from build123d import *

# Parameters (mm, degrees)
F1_DEPTH = 30
F2_T     = -5


with BuildPart() as f1:
    # F0 (on Top) → F1 (new body)
    with BuildSketch(Plane.XY):
        Polygon((0, 50), (-50, 0), (0, 0), align=None)
    extrude(amount=F1_DEPTH)

    # F2
    f2_openings = [f1.faces().sort_by_distance(p)[0] for p in [
        (-16.666667, 16.666667, 30),
    ]]
    offset(amount=F2_T, openings=f2_openings)


solid = f1.part
Verification items for the finished model (mm, model axes). A direction names the side the tool comes from. Coordinates: 2 decimals unless noted, no trailing zeros. Order: outer loops, then holes, each group sorted by start corner. A loop starts at its lowest first (then second) coordinate and runs counter-clockwise, first axis right, second up. Notation, with made-up numbers: (32.25, 29.25) -> (36.25, 29.25) arc R20 ccw to (36.25, 59.25) -> close; hole circle Ø3 at (33, 49). An arc over 180 degrees is marked (long way). Use CSV: the item, a comma, the result in double quotes. Start each with the question number.
Q1. Draft check along X on faces 1 (the flat face through (-14, 14, 5)), 2 (the flat face through (-23, 21, 30)), 3 (the flat face through (-25, 25, 15)). Enter one of: +X half, -X half, draft (parallel to the pull), parting line (faces both ways), or undercut.
Q2. Section check B-B, the plane x = -35.5. Record the cut outline in (y, z).
Q3. Section check A-A, the plane z = 28. Record the cut outline in (x, y), and give its area (3 significant figures).
Q4. Depth check by flat-ended pin: P1, Ø12.5, axis at y = 17, z = 19.5, coming from the -X side; P2, Ø7.5, axis at x = -14, z = 22.5, coming from the +Y side; P3, Ø2, axis at x = -28.5, z = 26.5, coming from the +Y side. Enter the tip coordinate at first touch or a pass-through.
Q5. Tool access check on faces 4 (the flat face through (-25, 0, 15)), 5 (the flat face through (-5, 21, 17)). Record the directions out of +Z, -Z, +X, -X, +Y, -Y that give a thin tool (end or side, any length) a straight path to the whole face; none if there is none.
Q6. Section check D-D, the plane z = 4.25. Record the cut outline in (x, y), and give its area (3 significant figures).
Q7. Section check C-C, the plane y = 26. Record the cut outline in (x, z), and give its area (3 significant figures).
Q8. Thickness scan on line 1 along Z through (x, y) = (-12, 26); line 2 along Y through (x, z) = (-23, 14); line 3 along X through (y, z) = (22.5, 15). Record the ranges inside material, lowest first.
Returned:
1,face 1,"undercut"
1,face 2,"draft"
1,face 3,"-X half"
2,outline,"(0, 0) -> (14.5, 0) -> (14.5, 30) -> (7.43, 30) -> (7.43, 5) -> (5, 5) -> (5, 30) -> (0, 30) -> close"
3,outline,"(-50, 0) -> (0, 0) -> (0, 50) -> close; hole (-37.93, 5) -> (-5, 5) -> (-5, 37.93) -> close"
3,area,"708 mm^2"
4,P1,"stops at x = -39.25"
4,P2,"stops at y = 39.75"
4,P3,"stops at y = 22.5"
5,face 4,"+Z, -Z, +X, -X, -Y"
5,face 5,"+Z"
6,outline,"(-50, 0) -> (0, 0) -> (0, 50) -> close"
6,area,"1,250 mm^2"
7,outline,"(-24, 0) -> (0, 0) -> (0, 30) -> (-5, 30) -> (-5, 5) -> (-16.93, 5) -> (-16.93, 30) -> (-24, 30) -> close"
7,area,"422 mm^2"
8,line 1,"z = 0 to 5"
8,line 2,"y = 0 to 5, 19.93 to 27"
8,line 3,"x = -27.5 to -20.43, -5 to 0"
